Model file for the job. Use its own axes, mm. A direction names the side the tool comes from. Round coordinates to 2 decimals unless told otherwise and drop trailing zeros. Loops run counter-clockwise (first coordinate to the right, second up) from the corner with the lowest first, then second, coordinate; pieces in that order, holes last. Notation, with made-up numbers: M -11.5,-6 L 22.5,-6 A11 ccw 22.5,-2 Z; hole C 27.5,83 d2. An arc over 180 degrees is marked long. Use a Markdown table: item, result. Add a question column.
Item 1: Saw through at D-D on x = 23. Write the cut outline in (y, z), then the cut area to 3 significant figures.
Item 2: Saw through at C-C on y = -17.5. Write the cut outline in (x, z).
Item 3: Wall check: L1, parallel to X at y = 0, z = 5.5; L2, parallel to Y at x = 0, z = 6.75; L3, parallel to X at y = -5, z = 9.5. Give the ranges that are in metal, low to high. Write a range as from..to.
Item 4: Saw through at A-A on y = 0. Write the cut outline in (x, z), then the cut area to 3 significant figures.
Item 5: Tool access for faces 1 (the flat face through (-27.94, 0, 10)), 2 (the flat face through (50.62, 17.01, 3.06)), 3 (the cylindrical face through (44.36, -1.03, 1.7)): list every direction of +Z, -Z, +X, -X, +Y, -Y with a clear straight run to the whole face (end or side of a thin tool).
Item 6: Two-plate mould, pull along X, no slides. Class faces 4 (the flat face through (38.1, -6, 6)), 5 (the flat face through (-6.35, -18, 10)), 6 (the flat face through (0, -18, 7.62)), 7 (the flat face through (-33, 0, 12.7)): +X half, -X half, draft (parallel to the pull), parting line (faces both ways), or undercut.
Item 7: Pin check, flat tips, straight feed: P1, Ø1.4, axis at x = -27.5, y = 5.5, coming from the +Z side; P2, Ø2.5, axis at y = -15, z = 10, coming from the +X side; P3, Ø2, axis at y = 3.5, z = 4.5, coming from the +X side; P4, Ø5.5, axis at x = 27, y = 7.5, coming from the +Z side. Stop position of each tip, or through.
Item 8: Saw through at B-B on x = 0. Write the cut outline in (y, z), then the cut area to 3 significant figures.
```python
from build123d import *

# Parameters (mm, degrees)
F0_W     = 76.2
F0_H     = 50.8
F0_R     = 12.7
F1_DEPTH = 12.7
F2_W     = 1.27
F2_H     = 50.8
F3_DEPTH = 5.08
F5_DEPTH = 50.801
F6_R     = 4.7625
F7_DEPTH = 12.7
F9_DEPTH = 25.4


with BuildPart() as f1:
    # F0 (on Top) → F1 (new body)
    with BuildSketch(Plane.XY):
        Rectangle(F0_W, F0_H)
        Circle(F0_R, mode=Mode.SUBTRACT)
    extrude(amount=F1_DEPTH)

    # F2 (on face) → F3 (cut)
    with BuildSketch(Plane.XY.offset(12.7)):
        with Locations((-27.305, 0)):
            Rectangle(F2_W, F2_H)
        with BuildLine():
            Line((-6.35, -10.9985226281), (-6.35, -25.4))
            Line((-6.35, -25.4), (6.35, -25.4))
            Line((6.35, -25.4), (6.35, -10.9985226281))
            ThreePointArc((6.35, -10.9985226281), (0, -12.7), (-6.35, -10.9985226281))
        make_face()
        with BuildLine():
            Line((6.35, 25.4), (-6.35, 25.4))
            Line((-6.35, 25.4), (-6.35, 10.9985226281))
            ThreePointArc((-6.35, 10.9985226281), (0, 12.7), (6.35, 10.9985226281))
            Line((6.35, 10.9985226281), (6.35, 25.4))
        make_face()
    extrude(amount=-F3_DEPTH, mode=Mode.SUBTRACT)

    # F4 (on face) → F5 (cut, through all)
    with BuildSketch(Plane.XZ.offset(25.4)):
        Polygon((31.75, 12.7), (19.05, 12.7), (16.1170606325, 7.62), (34.6829393675, 7.62), align=None)
    extrude(amount=-F5_DEPTH, mode=Mode.SUBTRACT)

    # F6 (on face) → F7 (join)
    with BuildSketch(Plane.YZ.offset(38.1)):
        with Locations((0, 6.35)):
            Circle(F6_R)
    extrude(amount=F7_DEPTH)

    # F8 (on face) → F9 (join)
    with BuildSketch(Plane.YZ.offset(38.1)):
        Polygon((12.2501304301, 12.7), (11.0074644908, 12.7), (14.1120990738, 0), (19.9945662171, 6.2075415626), (21.301779896, 0), (22.8132493794, 12.7), (21.8736864626, 12.7), (21.301779896, 5.513084121), (20.5153317719, 9.2476758682), (14.5206041634, 1.9182431279), align=None)
    extrude(amount=F9_DEPTH)


solid = f1.part
```
Entries:
| question | item | result |
|---|---|---|
| 1 | outline | M -25.4,0 L 25.4,0 L 25.4,7.62 L -25.4,7.62 Z |
| 1 | area | 387 mm2 |
| 2 | outline | M -38.1,0 L 38.1,0 L 38.1,12.7 L 31.75,12.7 L 34.68,7.62 L 16.12,7.62 L 19.05,12.7 L 6.35,12.7 L 6.35,7.62 L -6.35,7.62 L -6.35,12.7 L -26.67,12.7 L -26.67,7.62 L -27.94,7.62 L -27.94,12.7 L -38.1,12.7 Z |
| 3 | L1 | -38.1..-12.7, 12.7..50.8 |
| 3 | L2 | -25.4..-12.7, 12.7..25.4 |
| 3 | L3 | -38.1..-27.94, -26.67..-11.67, 11.67..17.2, 33.6..38.1 |
| 4 | outline | M -38.1,0 L -12.7,0 L -12.7,12.7 L -26.67,12.7 L -26.67,7.62 L -27.94,7.62 L -27.94,12.7 L -38.1,12.7 Z; M 12.7,0 L 38.1,0 L 38.1,1.59 L 50.8,1.59 L 50.8,11.11 L 38.1,11.11 L 38.1,12.7 L 31.75,12.7 L 34.68,7.62 L 16.12,7.62 L 19.05,12.7 L 12.7,12.7 Z |
| 4 | area | 680 mm2 |
| 5 | face 1 | +Z, +Y, -Y |
| 5 | face 2 | -Z, +X |
| 5 | face 3 | +X |
| 6 | face 4 | +X half |
| 6 | face 5 | undercut |
| 6 | face 6 | undercut |
| 6 | face 7 | draft |
| 7 | P1 | z = 12.7 |
| 7 | P2 | x = 38.1 |
| 7 | P3 | x = 50.8 |
| 7 | P4 | z = 7.62 |
| 8 | outline | M -25.4,0 L -12.7,0 L -12.7,7.62 L -25.4,7.62 Z; M 12.7,0 L 25.4,0 L 25.4,7.62 L 12.7,7.62 Z |
| 8 | area | 194 mm2 |
